from build123d import *

# Parameters (mm, degrees)
EXTRUDE1_DEPTH  = 110
LPATTERN1_COUNT = 3
LPATTERN1_PITCH = 60


with BuildPart() as part:
    # 15mm → Extrude1 (new, symmetric)
    with BuildSketch(Plane.XY):
        with BuildLine():
            Line((4.949972, 7.600006), (6.192321846, 7.599996))
            ThreePointArc((6.192321846, 7.599996), (6.706266371, 6.946742527), (7.49999, 6.7))
            Line((7.49999, 6.7), (7.49999, 1.000024142))
            Line((7.49999, 1.000024142), (6.499965858, 0))
            Line((6.499965858, 0), (-6.499965858, 0))
            Line((-6.499965858, 0), (-7.49999, 1.000024142))
            Line((-7.49999, 1.000024142), (-7.49999, 6.7))
            ThreePointArc((-7.49999, 6.7), (-6.70626637, 6.946742527), (-6.192321846, 7.599996))
            Line((-6.192321846, 7.599996), (-4.949982, 7.599996))
            Line((-4.949982, 7.599996), (-4.949972, 8.600006))
            Line((-4.949972, 8.600006), (-6.192326435, 8.600016))
            ThreePointArc((-6.192326435, 8.600016), (-6.706271662, 9.253261115), (-7.49999, 9.5))
            Line((-7.49999, 9.5), (-7.49999, 11.099974))
            ThreePointArc((-7.49999, 11.099974), (-6.510037425, 11.510033031), (-6.099989, 12.49999))
            Line((-6.099989, 12.49999), (6.099989, 12.49999))
            ThreePointArc((6.099989, 12.49999), (6.510037425, 11.510033031), (7.49999, 11.099974))
            Line((7.49999, 11.099974), (7.49999, 9.5))
            ThreePointArc((7.49999, 9.5), (6.706271662, 9.253261115), (6.192326435, 8.600016))
            Line((6.192326435, 8.600016), (4.949982, 8.600016))
            Line((4.949982, 8.600016), (4.949972, 7.600006))
        make_face()
    extrude(amount=EXTRUDE1_DEPTH, both=True)

    # Sketch1 → Cut-Revolve1 (revolve, cut)
    with BuildSketch(Plane(origin=(0, 0, 0), x_dir=(0, 0, -1), z_dir=(1, 0, 0))):
        Polygon((-90, 12.49999), (-86.25, 12.49999), (-86.25, 7.19999), (-87.75, 7.19999), (-87.75, 0), (-90, 0), align=None)
    revolve(axis=Axis((0, 0, 90), (0, 1, 0)), mode=Mode.SUBTRACT)

    # Sketch2 → Cut-Revolve2 (revolve, cut)
    with BuildSketch(Plane(origin=(0, 0, 0), x_dir=(0, 0, -1), z_dir=(1, 0, 0))):
        Polygon((90, 0), (92.25, 0), (92.25, 7.19999), (93.75, 7.19999), (93.75, 12.49999), (90, 12.49999), align=None)
    cut_revolve2 = revolve(axis=Axis((0, 12.49999, -90), (0, -1, 0)), mode=Mode.SUBTRACT)

    # LPattern1: Cut-Revolve2 ×3
    with Locations(*[(0, 0, i * LPATTERN1_PITCH) for i in range(1, LPATTERN1_COUNT)]):
        add(cut_revolve2, mode=Mode.SUBTRACT)


solid = part.part
Build history of the part. All positions in model axes, mm. A direction names the side the tool comes from. Round coordinates to 2 decimals unless told otherwise and drop trailing zeros. Loops run counter-clockwise (first coordinate to the right, second up) from the corner with the lowest first, then second, coordinate; pieces in that order, holes last. Notation, with made-up numbers: (-23.5, 23) -> (-11.5, 23) arc R19 cw to (-11.5, 27) -> close; hole circle Ø9 at (59, 76.25). An arc over 180 degrees is marked (long way). One line per item, written item: value. Start each with the question number.
Q1. Cut at A-A on z = 30. List the corners of the cut face in (x, y).
Q2. Drop flat-ended pins along their axis: pin 1 Ø4 at (x, z) = (1.5, 29.5) entering from +Y; pin 2 Ø1.1 at (y, z) = (8.5, 35) entering from +X; pin 3 Ø0.8 at (y, z) = (8.5, -46.5) entering from -X. Give the stop position or say it passes through.
Q3. Cut at C-C on x = 0. Count the separate pieces of the cut face and the enclosed holes in it, plus the area to 3 significant figures.
Q4. Two-plate mould, pull along X, no slides. Class faces 3 (the face through (7.5, 4, 2)), 4 (the face through (-7.5, 4, 2)), 5 (the face through (0, 6, -110)), 6 (the face through (1.436, 9.813, 86.536)): released by +X, released by -X, zero draft, split by the parting line, or undercut.
Q5. Probe line 1 along Z through (x, y) = (3, 11.25); line 2 along X through (y, z) = (4.25, 90); line 3 along Y through (x, z) = (-5.25, -36). List the from-to ranges inside material, lowest first.
Q6. 3-axis set-ups, long thin cutter, end or side, ignore diameter. For faces 1 (the face through (-0.86, 3.65, 27.92)), 2 (the face through (-1.436, 9.887, -93.464)): which of +Z, -Z, +X, -X, +Y, -Y reach the whole face in a straight line?
Q7. Cut at B-B on z = 67. List the corners of the cut face in (x, y).
Computed:
1. outline: (-7.5, 1) -> (-6.5, 0) -> (-2.25, 0) -> (-2.25, 7.2) -> (-3.75, 7.2) -> (-3.75, 12.5) -> (-6.1, 12.5) arc R1.4 cw to (-7.5, 11.1) -> (-7.5, 9.5) arc R1.4 cw to (-6.19, 8.6) -> (-4.95, 8.6) -> (-4.95, 7.6) -> (-6.19, 7.6) arc R1.4 cw to (-7.5, 6.7) -> close; (2.25, 0) -> (6.5, 0) -> (7.5, 1) -> (7.5, 6.7) arc R1.4 cw to (6.19, 7.6) -> (4.95, 7.6) -> (4.95, 8.6) -> (6.19, 8.6) arc R1.4 cw to (7.5, 9.5) -> (7.5, 11.1) arc R1.4 cw to (6.1, 12.5) -> (3.75, 12.5) -> (3.75, 7.2) -> (2.25, 7.2) -> close
2. pin 1: y = 7.2
2. pin 2: x = 6.47
2. pin 3: x = -6.35
3. separate pieces: 5
3. enclosed holes: 0
3. area: 2,460 mm²
4. face 3: released by +X
4. face 4: released by -X
4. face 5: zero draft
4. face 6: undercut
5. line 1: -110 to -92.25, -87.75 to -32.25, -27.75 to 27.75, 32.25 to 87.75, 92.25 to 110
5. line 2: -7.5 to -2.25, 2.25 to 7.5
5. line 3: 0 to 7.6, 8.6 to 12.5
6. face 1: +Y, -Y
6. face 2: +Y
7. outline: (-7.5, 1) -> (-6.5, 0) -> (6.5, 0) -> (7.5, 1) -> (7.5, 6.7) arc R1.4 cw to (6.19, 7.6) -> (4.95, 7.6) -> (4.95, 8.6) -> (6.19, 8.6) arc R1.4 cw to (7.5, 9.5) -> (7.5, 11.1) arc R1.4 cw to (6.1, 12.5) -> (-6.1, 12.5) arc R1.4 cw to (-7.5, 11.1) -> (-7.5, 9.5) arc R1.4 cw to (-6.19, 8.6) -> (-4.95, 8.6) -> (-4.95, 7.6) -> (-6.19, 7.6) arc R1.4 cw to (-7.5, 6.7) -> close
